The listing builds one solid part. Answer for the finished solid, in the listing's coordinates (mm). Face numbers are marked on the shaded views. A direction names the side the tool comes from. Round coordinates to 2 decimals unless told otherwise and drop trailing zeros. Write each loop counter-clockwise with the first axis right and the second up, starting at its lowest first coordinate (ties: lowest second). Pieces come first, ordered by that corner, then holes. Notation, with made-up numbers: M 40,39.25 L 54,39.25 A29 cw 54,70.25 Z; hole C -40,79.5 d9. An arc over 180 degrees is marked long. One line per item, written item: value. Start each with the question number.
(1) Consider probe 1 along X at (y, z) = (5, 165) (3 decimals); probe 2 along Z at (x, y) = (-284, 313) (3 decimals). Determine where each line is inside the solid, lowest interval first.
(2) Given P1, Ø8, axis at x = 129.5, y = 201, coming from the +Z side (3 decimals); P2, Ø12, axis at x = -112.5, y = -316, coming from the -Z side; P3, Ø9.5, axis at x = -438.5, y = -441, coming from the +Z side (3 decimals), each flat-ended and moving along its own axis, determine where each tip first touches the part or whether it passes through.
(3) For the marked faces 4 and 5, determine the directions among +Z, -Z, +X, -X, +Y, -Y from which every point of the face is accessible in a straight line to the end or side of a thin tool.
(4) Section B-B (y = -359) is taken. Determine the outline of the cut face in (x, z) (3 decimals), plus the area to 3 significant figures.
(5) For a pull along Y with two mould halves and no side action, classify the marked faces 1, 2 and 3 as released by +Y, released by -Y, zero draft, split by the parting line, or undercut.
(6) Section A-A (z = 177.5) is taken. Determine the outline of the cut face in (x, y) (3 decimals), plus the area to 3 significant figures.
```python
from build123d import *

# Parameters (mm, degrees)
F0_W     = 914.4
F0_H     = 914.4
F1_DEPTH = 3.175
F2_W     = 914.4
F2_H     = 914.4
F2_W_2   = 908.05
F2_H_2   = 908.05
F3_DEPTH = 203.2
F4_W     = 38.1
F4_H     = 38.1
F5_DEPTH = 50.8
F6_T     = -3.175


with BuildPart() as f1:
    # F0 (on Top) → F1 (new body)
    with BuildSketch(Plane.XY):
        Rectangle(F0_W, F0_H)
    extrude(amount=F1_DEPTH)

    # F2 (on face) → F3 (join)
    with BuildSketch(Plane.XY.offset(3.175)):
        Rectangle(F2_W, F2_H)
        Rectangle(F2_W_2, F2_H_2, mode=Mode.SUBTRACT)
        Rectangle(F2_W_2, F2_H_2)
    extrude(amount=F3_DEPTH)

    # F4 (on face) → F5 (join)
    with BuildSketch(Plane(origin=(0, 0, 0), x_dir=(1, 0, 0), z_dir=(0, 0, -1))):
        with Locations((-438.15, -438.15)):
            Rectangle(F4_W, F4_H)
        with Locations((438.15, -438.15)):
            Rectangle(F4_W, F4_H)
        with Locations((438.15, 438.15)):
            Rectangle(F4_W, F4_H)
        with Locations((-438.15, 438.15)):
            Rectangle(F4_W, F4_H)
    extrude(amount=F5_DEPTH)

    # F6
    f6_openings = [f1.faces().sort_by_distance(p)[0] for p in [
        (0, 0, 206.375),
    ]]
    offset(amount=F6_T, openings=f6_openings, kind=Kind.INTERSECTION)


solid = f1.part
```
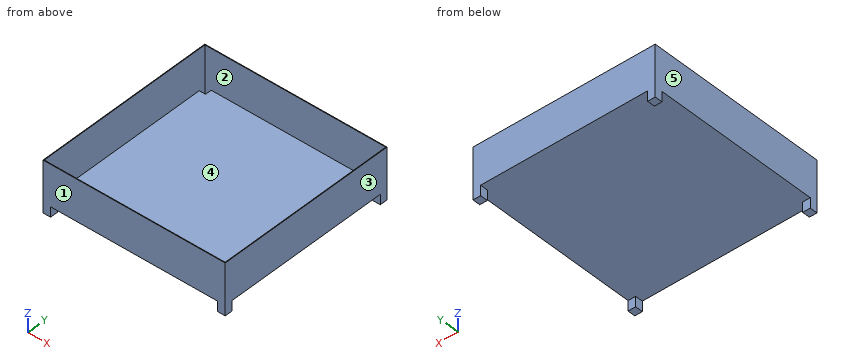
Recorded:
1. probe 1: x = -457.2 to -454.025, 454.025 to 457.2
1. probe 2: z = 0 to 3.175
2. P1: stops at z = 3.175
2. P2: stops at z = 0
2. P3: stops at z = -47.625
3. face 4: +Z
3. face 5: +Z, -Z, -X, +Y, -Y
4. outline: M -457.2,0 L 457.2,0 L 457.2,206.375 L 454.025,206.375 L 454.025,3.175 L -454.025,3.175 L -454.025,206.375 L -457.2,206.375 Z
4. area: 4,190 mm2
5. face 1: released by -Y
5. face 2: undercut
5. face 3: zero draft
6. outline: M -457.2,-457.2 L 457.2,-457.2 L 457.2,457.2 L -457.2,457.2 Z; hole M -454.025,-454.025 L 454.025,-454.025 L 454.025,454.025 L -454.025,454.025 Z
6. area: 11,600 mm2
